Study the drawing (mm; zero at the part's minimum x, y, z) and answer. Give positions to 0.01 mm unless a question says otherwise; leave off trailing zeros. Order: outer loops, then holes, each group sorted by start corner. A loop starts at its lowest first (then second) coordinate and runs counter-clockwise, first axis right, second up. Notation, with made-up numbers: (39, 81.25) -> (50, 81.25) arc R21 ccw to (50, 114.25) -> close; hole circle Ø5 at (76, -28.5). An arc over 180 degrees is marked (long way). Answer as CSV lines item,"result". Start each with the question number.
1. A cutting plane is placed at A-A (z = 2.05). Give the vertices of the cut face in (x, y) (1 decimal).
2. A flat-ended cylindrical pin translates along its axis: pin 1 (1 mm diameter, centred on x = 2, z = 1.5, fed in from -Y). Find the tip coordinate at first contact, or state that the pin passes through.
3. A cutting plane is placed at D-D (y = 4). Give the vertices of the cut face in (x, z), then the cut area to 3 significant figures.
4. Find the intervals of material crossed by L1, parallel to Y at x = 7.5, z = 1.85 (1 decimal); L2, parallel to X at y = 8.5, z = 2.55 (1 decimal); L3, parallel to X at y = 8.75, z = 2.5 (1 decimal), in increasing order.
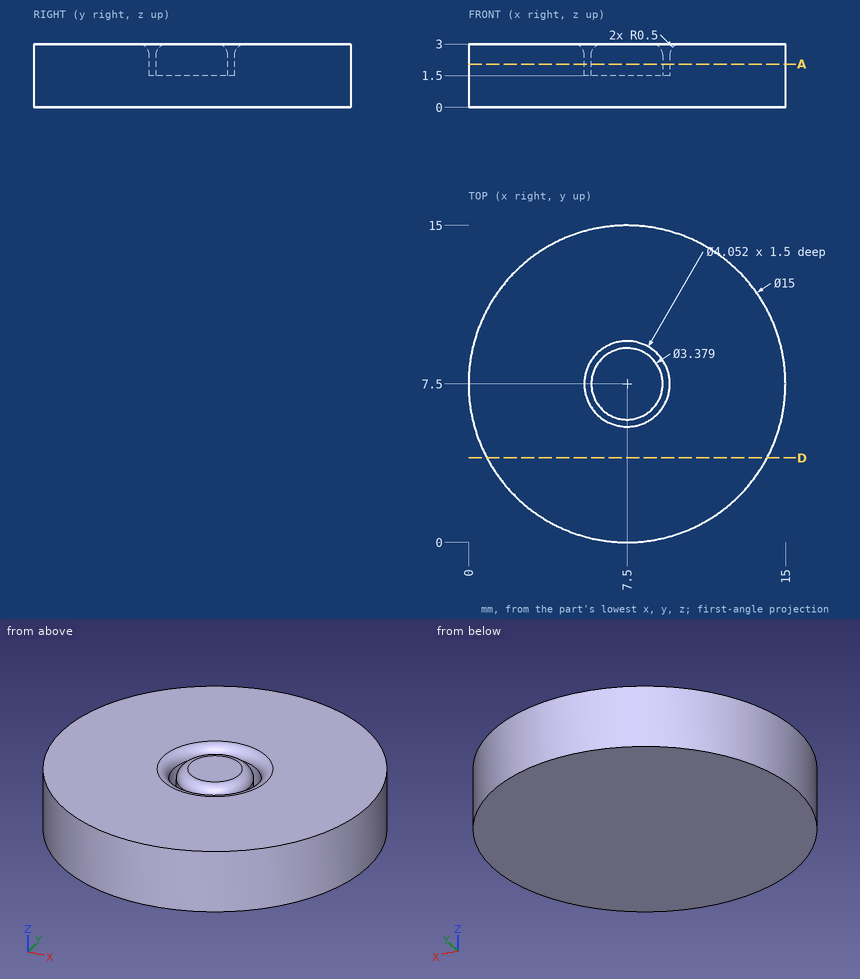
Answer sheet:
1,outline,"circle Ø15 at (7.5, 7.5); circle Ø3.4 at (7.5, 7.5); hole circle Ø4.1 at (7.5, 7.5)"
2,pin 1,"stops at y = 1.91"
3,outline,"(0.87, 0) -> (14.13, 0) -> (14.13, 3) -> (0.87, 3) -> close"
3,area,"39.8 mm^2"
4,L1,"y = 0 to 5.5, 5.8 to 9.2, 9.5 to 15"
4,L2,"x = 0.1 to 5.7, 6.1 to 8.9, 9.3 to 14.9"
4,L3,"x = 0.1 to 5.9, 6.4 to 8.6, 9.1 to 14.9"
